from build123d import *

# Parameters (mm, degrees)
ESQUISSE1_W        = 128.24605794
ESQUISSE1_H        = 10
BOSS_EXTRU_2_DEPTH = 2
ESQUISSE2_W        = 128.24605794
ESQUISSE2_H        = 2
BOSS_EXTRU_3_DEPTH = 24
ESQUISSE3_W        = 128.24605794
ESQUISSE3_H        = 8
BOSS_EXTRU_4_DEPTH = 2


with BuildPart() as part:
    # Esquisse1 → Boss.-Extru.2 (new body)
    with BuildSketch(Plane.XY):
        with Locations((-64.12703781, 124.040016289)):
            Rectangle(ESQUISSE1_W, ESQUISSE1_H)
    extrude(amount=BOSS_EXTRU_2_DEPTH)

    # Esquisse2 → Boss.-Extru.3 (add)
    with BuildSketch(Plane.XY.offset(2)):
        with Locations((-64.12703781, 128.040016289)):
            Rectangle(ESQUISSE2_W, ESQUISSE2_H)
    extrude(amount=BOSS_EXTRU_3_DEPTH)

    # Esquisse3 → Boss.-Extru.4 (add)
    with BuildSketch(Plane.XY.offset(26)):
        with Locations((-64.12703781, 125.040016289)):
            Rectangle(ESQUISSE3_W, ESQUISSE3_H)
    extrude(amount=BOSS_EXTRU_4_DEPTH)


solid = part.part
Work out the finished part from the listing and answer in its coordinate system (mm). A direction names the side the tool comes from. Coordinates: 2 decimals unless noted, no trailing zeros. Loops run counter-clockwise (first coordinate to the right, second up) from the corner with the lowest first, then second, coordinate; pieces in that order, holes last. Notation, with made-up numbers: M -5,-22.75 L 6,-22.75 A28 cw 6,4.25 Z; hole C -36,28.5 d10. An arc over 180 degrees is marked long. Answer in a Markdown table with one row per item. Add a question column.
1. Find section A-A, the plane y = 124.25. Write down the section's boundary in (x, z).
2. Find section B-B, the plane x = -32.5. Write down the section's boundary in (y, z), then the cut area to 3 significant figures.
3. The mould has two halves that part along Z. Classify faces 1 (the flat face through (-65, 124, 26)), 2 (the flat face through (-65, 125, 28)), 3 (the flat face through (-128.25, 127.3, 13.8)): pulls with the +Z half, pulls with the -Z half, needs draft (parallel to the pull), parting line crosses it, or undercut.
4. Find section C-C, the plane z = 19.75. Write down the section's boundary in (x, y), then the cut area to 3 significant figures.
5. Flat-ended cylindrical pins translate along their axes: P1, Ø5, axis at x = -91.5, z = 3.5, coming from the -Y side; P2, Ø2, axis at x = -76, z = 27.5, coming from the -Y side; P3, Ø3, axis at x = -23, z = 6.5, coming from the -Y side. Find the tip coordinate at first contact, or state that the pin passes through.
6. A tool of negligible diameter and unlimited length cuts with its end or side. For faces 4 (the flat face through (-65, 127.04, 14)), 5 (the flat face through (-65, 129.04, 14)), 6 (the flat face through (-65, 121.04, 27)), from which of +Z, -Z, +X, -X, +Y, -Y can it reach the whole face along a straight path? Write none if from no direction.
7. Consider L1, parallel to Z at x = -56, y = 124.5; L2, parallel to Z at x = -14.5, y = 120; L3, parallel to Y at x = -40, z = 25.75. Determine where each line is inside the solid, lowest interval first.
Reported:
| question | item | result |
|---|---|---|
| 1 | outline | M -128.25,0 L 0,0 L 0,2 L -128.25,2 Z; M -128.25,26 L 0,26 L 0,28 L -128.25,28 Z |
| 2 | outline | M 119.04,0 L 129.04,0 L 129.04,28 L 121.04,28 L 121.04,26 L 127.04,26 L 127.04,2 L 119.04,2 Z |
| 2 | area | 84.0 mm^2 |
| 3 | face 1 | undercut |
| 3 | face 2 | pulls with the +Z half |
| 3 | face 3 | needs draft |
| 4 | outline | M -128.25,127.04 L 0,127.04 L 0,129.04 L -128.25,129.04 Z |
| 4 | area | 256 mm^2 |
| 5 | P1 | stops at y = 119.04 |
| 5 | P2 | stops at y = 121.04 |
| 5 | P3 | stops at y = 127.04 |
| 6 | face 4 | +X, -X, -Y |
| 6 | face 5 | +Z, -Z, +X, -X, +Y |
| 6 | face 6 | +Z, +X, -X, -Y |
| 7 | L1 | z = 0 to 2, 26 to 28 |
| 7 | L2 | z = 0 to 2 |
| 7 | L3 | y = 127.04 to 129.04 |
